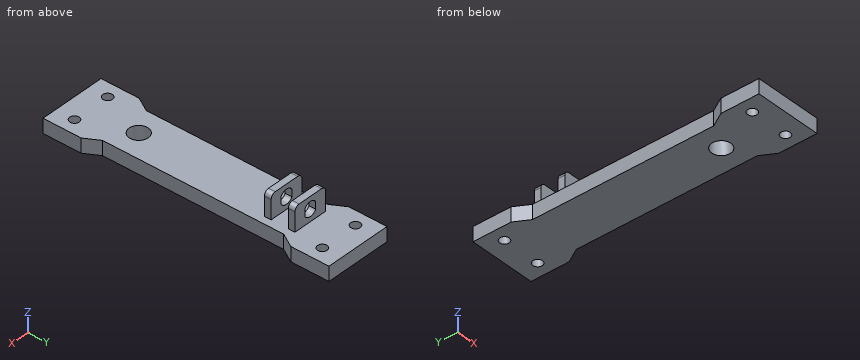
from build123d import *

# Parameters (mm, degrees)
BOSS_EXTRUDE1_DEPTH = 15
SKETCH3_R           = 5
CUT_EXTRUDE1_DEPTH  = 155.757875405
SKETCH4_R           = 10
CUT_EXTRUDE2_DEPTH  = 155.757875405
SKETCH6_W           = 37
SKETCH6_H           = 7
BOSS_EXTRUDE2_DEPTH = 25
CUT_EXTRUDE3_DEPTH  = 32
FILLET3_R           = 5


with BuildPart() as part:
    # Sketch2 → Boss-Extrude1 (new body)
    with BuildSketch(Plane.XY):
        Polygon((-35, 110), (-26.339745962, 95), (-26.339745962, -95), (-35, -110), (-35, -150), (35, -150), (35, -110), (26.339745962, -95), (26.339745962, 95), (35, 110), (35, 150), (-35, 150), align=None)
    extrude(amount=BOSS_EXTRUDE1_DEPTH)

    # Sketch3 → Cut-Extrude1 (cut, through all)
    with BuildSketch(Plane.XY.offset(15)):
        with Locations((-20, 130)):
            Circle(SKETCH3_R)
        with Locations((20, 130)):
            Circle(SKETCH3_R)
        with Locations(Location((20, -130, 0), (0, 0, 180))):
            Circle(SKETCH3_R)
        with Locations(Location((-20, -130, 0), (0, 0, 180))):
            Circle(SKETCH3_R)
    extrude(amount=-CUT_EXTRUDE1_DEPTH, mode=Mode.SUBTRACT)

    # Sketch4 → Cut-Extrude2 (cut, through all)
    with BuildSketch(Plane.XY.offset(15)):
        with Locations((0, -80)):
            Circle(SKETCH4_R)
    extrude(amount=-CUT_EXTRUDE2_DEPTH, mode=Mode.SUBTRACT)

    # Sketch6 → Boss-Extrude2 (add)
    with BuildSketch(Plane.XY.offset(15)):
        with Locations((0, 96.5)):
            Rectangle(SKETCH6_W, SKETCH6_H)
        with Locations((0, 71.5)):
            Rectangle(SKETCH6_W, SKETCH6_H)
    extrude(amount=BOSS_EXTRUDE2_DEPTH)

    # Sketch7 → Cut-Extrude3 (cut)
    with BuildSketch(Plane.XZ.offset(-68)):
        with BuildLine():
            Line((-6.5, 31.241657387), (-6.5, 23.758342613))
            ThreePointArc((-6.5, 23.758342613), (0, 20), (6.5, 23.758342613))
            Line((6.5, 23.758342613), (6.5, 31.241657387))
            ThreePointArc((6.5, 31.241657387), (0, 35), (-6.5, 31.241657387))
        make_face()
    extrude(amount=-CUT_EXTRUDE3_DEPTH, mode=Mode.SUBTRACT)

    # Fillet3
    fillet3_edges = [part.edges().sort_by_distance(p)[0] for p in [
        (18.5, 96.5, 40),
        (-18.5, 96.5, 40),
        (18.5, 71.5, 40),
        (-18.5, 71.5, 40),
    ]]
    fillet(fillet3_edges, radius=FILLET3_R)


solid = part.part
Could you check a few things on this model? Use its own coordinates, in mm. Coordinates: 2 decimals unless noted, no trailing zeros. Loops run counter-clockwise (first coordinate to the right, second up) from the corner with the lowest first, then second, coordinate; pieces in that order, holes last.
1. Imagine slicing it at D-D (y = -130). Please give me the cut outline in (x, z), and give its area (3 significant figures).
2. For P1, Ø5.5, axis at y = 97, z = 26.5, coming from the +X side; P2, Ø6, axis at x = 10, y = -48, coming from the -Z side; P3, Ø12.5, axis at x = 3, z = 25.5, coming from the +Y side; P4, Ø4, axis at x = 15, y = 78.5, coming from the +Z side, each with a flat end and sliding along its axis, tell me the tip position at first contact or that it passes through.
3. I need wall thicknesses on L1, parallel to X at y = -130, z = 4; L2, parallel to Y at x = 20, z = 11.75; L3, parallel to Y at x = 17, z = 34.5. Which ranges of each line are inside material? Lowest first, please.
4. Imagine slicing it at B-B (z = 27.5). Please give me the cut outline in (x, y), and give its area (3 significant figures).
5. Imagine slicing it at A-A (y = -80). Please give me the cut outline in (x, z).
6. Imagine slicing it at C-C (x = 0). Please give me the cut outline in (y, z), and give its area (3 significant figures).
Computed values:
1. outline: (-35, 0) - (-25, 0) - (-25, 15) - (-35, 15) - close; (-15, 0) - (15, 0) - (15, 15) - (-15, 15) - close; (25, 0) - (35, 0) - (35, 15) - (25, 15) - close
1. area: 750 mm2
2. P1: stops at x = 18.5
2. P2: stops at z = 0
2. P3: stops at y = 100
2. P4: stops at z = 15
3. L1: x = -35 to -25, -15 to 15, 25 to 35
3. L2: y = -150 to -135, -125 to 125, 135 to 150
3. L3: y = 68 to 75, 93 to 100
4. outline: (-18.5, 68) - (-6.5, 68) - (-6.5, 75) - (-18.5, 75) - close; (-18.5, 93) - (-6.5, 93) - (-6.5, 100) - (-18.5, 100) - close; (6.5, 68) - (18.5, 68) - (18.5, 75) - (6.5, 75) - close; (6.5, 93) - (18.5, 93) - (18.5, 100) - (6.5, 100) - close
4. area: 336 mm2
5. outline: (-26.34, 0) - (-10, 0) - (-10, 15) - (-26.34, 15) - close; (10, 0) - (26.34, 0) - (26.34, 15) - (10, 15) - close
6. outline: (-150, 0) - (-90, 0) - (-90, 15) - (-150, 15) - close; (-70, 0) - (150, 0) - (150, 15) - (100, 15) - (100, 20) - (93, 20) - (93, 15) - (75, 15) - (75, 20) - (68, 20) - (68, 15) - (-70, 15) - close; (68, 35) - (75, 35) - (75, 40) - (68, 40) - close; (93, 35) - (100, 35) - (100, 40) - (93, 40) - close
6. area: 4,340 mm2
